Check sheet for the modelled part. Datum: model origin and axes. Units: mm. A direction names the side the tool comes from. Give positions to 0.01 mm unless a question says otherwise; leave off trailing zeros. Order: outer loops, then holes, each group sorted by start corner. A loop starts at its lowest first (then second) coordinate and runs counter-clockwise, first axis right, second up.
Autodesk Inventor part; units mm, degrees
ref_plane "YZ Plane" through (0, 0, 0) normal (1, 0, 0) x (0, 1, 0)
ref_plane "XZ Plane" through (0, 0, 0) normal (0, 1, 0) x (-1, 0, 0)
ref_plane "XY Plane" through (0, 0, 0) normal (0, 0, 1) x (1, 0, 0)
sketch "Sketch1" plane through (0, 0, 0) normal (0, 0, 1) x (1, 0, 0)
  line L0 (0, 17.0681) -> (0, -16.825)
  line L1 (2, 2.3018) -> (2, -2.3018)
  line L2 (2, -2.3018) -> (8.5, -2.3018)
  line L3 (8.5, -2.3018) -> (8.5, -4.5)
  line L4 (8.5, -4.5) -> (12.5, -4.5)
  line L5 (12.5, -4.5) -> (12.5, 4.5)
  line L6 (12.5, 4.5) -> (8.5, 4.5)
  line L7 (8.5, 4.5) -> (8.5, 2.3018)
  line L8 (8.5, 2.3018) -> (2, 2.3018)
  line L9 (12.5, 3) -> (10.5, 1.8453)
  line L10 (10.5, 1.8453) -> (10.5, -1.8453)
  line L11 (10.5, -1.8453) -> (12.5, -3)
  point P0 (0, 0)
  point P1 (0, 0.1215)
  point P2 (2, 0)
  dimension "d0" = 25
  dimension "d1" = 4
  dimension "d2" = 4
  dimension "d3" = 9
  dimension "d4" = 1.5
  dimension "d5" = 1.5
  dimension "d6" = 2
  dimension "d7" = 60
revolve "Revolution1" add sketch "Sketch1" angle 360 about axis through (0, 17.0681, 0) along (0, -1, 0) contours L8 L7 L6 L5 L9 L10 L11 L4 L3 L2 L1
sketch "Sketch2" plane through (0, -2.3018, 0) normal (0, -1, 0) x (1, 0, 0)
  circle A0 centre (0, 0) radius 2 construction
  circle A1 centre (0, 0) radius 5 construction
  circle A2 centre (-5, 0) radius 2
  circle A3 centre (-1.5451, -4.7553) radius 2
  circle A4 centre (4.0451, -2.9389) radius 2
  circle A5 centre (4.0451, 2.9389) radius 2
  circle A6 centre (-1.5451, 4.7553) radius 2
  point P0 (0, 0)
  dimension "d9" = 10
  dimension "d10" = 4
  dimension "d13" = 360
extrude "Extrusion1" cut sketch "Sketch2" against normal through all
sketch "Sketch3" plane through (0, 2.3018, 0) normal (0, 1, 0) x (1, 0, 0)
  circle A0 centre (0, 0) radius 2.5
  circle A1 centre (0, 0) radius 2
  point P0 (0, 0)
  dimension "d17" = 5
extrude "Extrusion2" add sketch "Sketch3" along normal blind 0.5
mirror "Mirror1" about plane through (0, 0, 0) normal (0, 1, 0) of "Extrusion2"
fillet "Fillet1" radius 0.2 1 edges at (-2.5, 2.3018, 0)
fillet "Fillet2" radius 0.2 1 edges at (-2.5, -2.3018, 0)
fillet "Fillet3" radius 0.1 2 edges at (-2, 2.8018, 0) (-2, -2.8018, 0)
properties part number "Pulley nhỏ" material "Iron, Cast"
1) Section check A-A, the plane y = 1.25. Record the cut outline in (x, z), then the cut area to 3 significant figures.
Recorded:
outline: circle Ø21 at (0, 0); hole circle Ø4 at (-5, 0); hole circle Ø4 at (-1.55, -4.76); hole circle Ø4 at (-1.55, 4.76); hole circle Ø4 at (0, 0); hole circle Ø4 at (4.05, -2.94); hole circle Ø4 at (4.05, 2.94)
area: 271 mm2
2) Section check B-B, the plane z = 0. State how many separate pieces and enclosed holes the cut face has, then the cut area to 3 significant figures.
Recorded:
separate pieces: 3
enclosed holes: 0
area: 95.1 mm2
3) Set-up check for faces 5 (the face through (10, 2, 4)), 6 (the face through (4.57, 3.386, 7.167)), 7 (the face through (4.57, -3.416, 7.167)): record each of +Z, -Z, +X, -X, +Y, -Y from which the full face is reachable in a straight line by a thin tool's end or side.
Recorded:
face 5: none
face 6: +Y
face 7: -Y
4) Draft check along Z on faces 1 (the face through (-3, 4.5, -8.2)), 2 (the face through (0, 0, -2)), 3 (the face through (11.923, -3.74, -3.755)), 4 (the face through (4, 2.302, 0)). Enter one of: +Z half, -Z half, draft (parallel to the pull), parting line (faces both ways), or undercut.
Recorded:
face 1: draft
face 2: undercut
face 3: parting line
face 4: undercut
5) Material ranges on L1, parallel to X at y = 0.75, z = 3.25; L2, parallel to Z at x = 0, y = -2.75; L3, parallel to X at y = 0.25, z = -1.5, recorded low to high.
Recorded:
L1: x = -9.98 to -2.86, -0.23 to 2.07, 6.02 to 9.98
L2: z = -12.07 to -8.5, -2.5 to -2.01, 2.01 to 2.5, 8.5 to 12.07
L3: x = -10.39 to -6.32, -3.68 to -1.32, 1.32 to 2.66, 5.43 to 10.39
6) Depth check by flat-ended pin: pin 1 Ø5 at (x, z) = (0.5, 3) entering from -Y; pin 2 Ø1.5 at (x, z) = (0, 1) entering from +Y; pin 3 Ø5 at (x, z) = (0, 0.5) entering from +Y; pin 4 Ø1 at (y, z) = (-0.5, 4) entering from -X. Enter the tip coordinate at first touch or a pass-through.
Recorded:
pin 1: stops at y = -2.8
pin 2: passes through
pin 3: stops at y = 2.8
pin 4: stops at x = -9.9
